Source: CAD feature listing. Evaluate the final solid. Frame: model axes, mm. Give positions to 0.01 mm unless a question says otherwise; leave off trailing zeros. Write each loop counter-clockwise with the first axis right and the second up, starting at its lowest first coordinate (ties: lowest second). Pieces come first, ordered by that corner, then holes.
```python
from build123d import *

# Parameters (mm, degrees)
SKETCH_2_R          = 0.975
EXTRUDE_1_DEPTH     = 28
EXTRUDE_2_DEPTH     = 23.8
SKETCH_5_R          = 0.975
EXTRUDE_3_DEPTH     = 2
CUT_EXTRUDE_START   = -2
SKETCH_7_R          = 2.125
CUT_EXTRUDE_1_DEPTH = 2
CHAMFER_1_SIZE      = 0.5
CHAMFER_2_SIZE      = 0.5
CHAMFER_3_SIZE      = 0.5
CHAMFER_4_SIZE      = 0.5
CHAMFER_7_SIZE      = 0.2


with BuildPart() as part:
    # 草图2 → 凸台-拉伸1 (new body)
    with BuildSketch(Plane(origin=(0, 0, 0), x_dir=(1, 0, 0), z_dir=(0, 1, 0))):
        with Locations(Location((0, 0, 0), (0, 0, 270))):
            Circle(SKETCH_2_R)
    extrude(amount=EXTRUDE_1_DEPTH)

    # 草图4 → 凸台-拉伸2 (add)
    with BuildSketch(Plane(origin=(0, 28, 0), x_dir=(1, 0, 0), z_dir=(0, 1, 0))):
        with BuildLine():
            Line((0, -48.5), (-2.125, -48.5))
            Line((-2.125, -48.5), (-2.125, 0))
            ThreePointArc((-2.125, 0), (0, 2.125), (2.125, 0))
            Line((2.125, 0), (2.125, -47.7))
            Line((2.125, -47.7), (2.125, -50.625))
            Line((2.125, -50.625), (0, -50.625))
            Line((0, -50.625), (0, -48.5))
        make_face()
    extrude(amount=-EXTRUDE_2_DEPTH)

    # 草图5 → 凸台-拉伸3 (add)
    with BuildSketch(Plane(origin=(0, 28, 0), x_dir=(1, 0, 0), z_dir=(0, 1, 0))):
        with Locations(Location((0, 0, 0), (0, 0, 270))):
            Circle(SKETCH_5_R)
    extrude(amount=EXTRUDE_3_DEPTH)

    # 草图7 → 切除-拉伸1 (cut)
    with BuildSketch(Plane.XZ.offset(CUT_EXTRUDE_START)):
        Circle(SKETCH_7_R)
    extrude(amount=CUT_EXTRUDE_1_DEPTH, mode=Mode.SUBTRACT)

    # 倒角1
    chamfer_1_edges = [part.edges().sort_by_distance(p)[0] for p in [
        (2.125, 28, 25.3125),
        (0, 28, -2.125),
        (-2.125, 28, 24.25),
        (-2.125, 4.2, 24.25),
        (0, 4.2, -2.125),
        (2.125, 4.2, 25.3125),
    ]]
    chamfer(chamfer_1_edges, length=CHAMFER_1_SIZE)

    # 倒角2
    chamfer_2_edges = [part.edges().sort_by_distance(p)[0] for p in [
        (-2.125, 16.1, 48.5),
        (2.125, 16.1, 50.625),
    ]]
    chamfer(chamfer_2_edges, length=CHAMFER_2_SIZE)

    # 倒角3
    chamfer_3_edges = [part.edges().sort_by_distance(p)[0] for p in [
        (0, 16.1, 50.625),
        (0, 16.1, 48.5),
    ]]
    chamfer(chamfer_3_edges, length=CHAMFER_3_SIZE)

    # 倒角4
    chamfer_4_edges = [part.edges().sort_by_distance(p)[0] for p in [
        (-1.0625, 28, 48.5),
        (-1.0625, 4.2, 48.5),
        (0, 28, 49.5625),
        (0, 4.2, 49.5625),
        (1.0625, 28, 50.625),
        (0.25, 28, 50.375),
        (1.0625, 4.2, 50.625),
        (0.25, 4.2, 50.375),
        (-0.25, 28, 48.75),
        (-0.25, 4.2, 48.75),
    ]]
    chamfer(chamfer_4_edges, length=CHAMFER_4_SIZE)

    # 倒角7
    chamfer_7_edges = [part.edges().sort_by_distance(p)[0] for p in [
        (0, 30, -0.975),
        (0, 2, -0.975),
    ]]
    chamfer(chamfer_7_edges, length=CHAMFER_7_SIZE)


solid = part.part
```
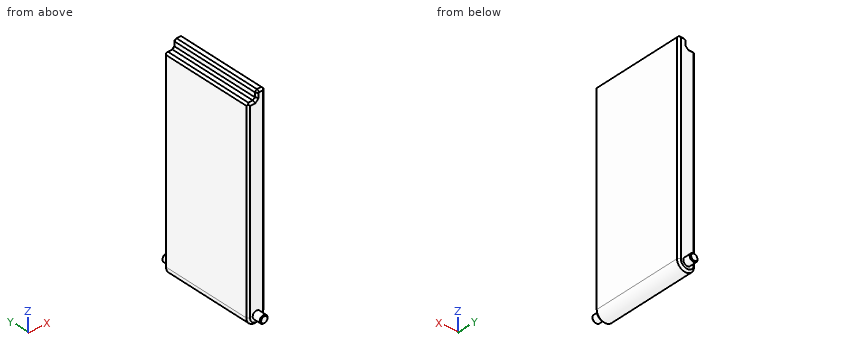
1. Line query: probe 1 along Y at (x, z) = (-0.95, 43); probe 2 along Z at (x, y) = (-0.2, 10.25); probe 3 along Y at (x, z) = (1.9, 19) (3 decimals). Output: solid intervals per line, ascending.
2. Pin query (flat end, axial travel): P1, Ø0.9, axis at y = 16.5, z = 49.5, coming from the -X side; P2, Ø0.6, axis at x = -1, y = 19.5, coming from the +Z side; P3, Ø1.5, axis at x = -0.5, y = 18, coming from the +Z side (3 decimals). Return the tip coordinate at first contact, or that it passes through.
3. Section query B-B (z = 12.5). Return loops of the section in (x, y) (3 decimals), plus the area to 3 significant figures.
4. Section query A-A (y = 13). Return loops of the section in (x, z) (3 decimals).
The answers:
1. probe 1: y = 4.2 to 28
1. probe 2: z = -2.12 to 48.8
1. probe 3: y = 4.475 to 27.725
2. P1: stops at x = 0
2. P2: stops at z = 48.5
2. P3: stops at z = 50.375
3. outline: (-2.125, 4.7) - (-1.625, 4.2) - (1.625, 4.2) - (2.125, 4.7) - (2.125, 27.5) - (1.625, 28) - (-1.625, 28) - (-2.125, 27.5) - close
3. area: 101 mm2
4. outline: (-2.125, 0) arc R2.125 ccw to (2.125, 0) - (2.125, 50.125) - (1.625, 50.625) - (0.5, 50.625) - (0, 50.125) - (0, 49) - (-0.5, 48.5) - (-1.625, 48.5) - (-2.125, 48) - close
